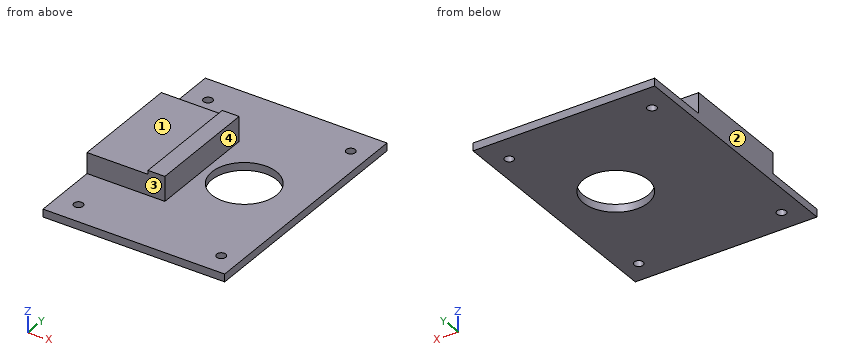
Autodesk Fusion 360 part; units mm, degrees
sketch "Sketch1" plane through (0, 0, 0) normal (0, 0, 1) x (1, 0, 0)
  line L0 (0, 0) -> (70, 0)
  line L1 (70, 0) -> (70, 54)
  line L2 (70, 54) -> (0, 54)
  line L3 (0, 54) -> (0, 0)
  line L4 (0, 0) -> (70, 0)
  line L5 (70, 0) -> (70, -20)
  line L6 (70, -20) -> (0, -20)
  line L7 (0, -20) -> (0, 0)
  line L8 (0, 54) -> (70, 54)
  line L9 (70, 54) -> (70, 74)
  line L10 (70, 74) -> (0, 74)
  line L11 (0, 74) -> (0, 54)
  dimension "d1" = 54
  dimension "d2" = 70
  dimension "d3" = 20
  dimension "d4" = 20
extrude "Extrude1" add sketch "Sketch1" along normal blind 3
hole "Hole1" at (45.2511, 28.5377, 3) direction (0, 0, -1) diameter 25 depth 5 tip angle 180
sketch "Sketch3" plane through (0, 0, 3) normal (0, 0, 1) x (-1, 0, 0)
  circle A0 centre (-45.2511, -28.5377) radius 12.5
  line L0 (0, -48.5) -> (-30.0019, -48.5)
  line L1 (-30.0019, -48.5) -> (-30.0019, -5.5)
  line L2 (-30.0019, -5.5) -> (0, -5.5)
  line L3 (0, -5.5) -> (0, -48.5)
  line L4 (-70, 20) -> (-70, -74)
  line L5 (-70, -74) -> (0, -74)
  line L6 (0, -74) -> (0, 20)
  line L7 (0, 20) -> (-70, 20)
  dimension "d20" = 25.5
  dimension "d21" = 25.5
extrude "Extrude3" add sketch "Sketch3" along normal blind 8 contours L0 L1 L2 L3 L6
sketch "Sketch4" plane through (0, 0, 3) normal (0, 0, 1) x (-1, 0, 0)
  line L0 (0, -48.5) -> (-30.0019, -48.5)
  line L1 (-30.0019, -48.5) -> (-30.0019, -5.5)
  line L2 (-30.0019, -5.5) -> (0, -5.5)
  line L3 (0, -5.5) -> (0, 20)
  line L4 (0, 20) -> (-70, 20)
  line L5 (-70, 20) -> (-70, -74)
  line L6 (-70, -74) -> (0, -74)
  line L7 (0, -74) -> (0, -48.5)
  circle A0 centre (-45.2511, -28.5377) radius 12.5
  circle A1 centre (-8, -63.531) radius 1.75
  circle A2 centre (-63, -63.531) radius 1.75
  circle A3 centre (-8, 11.469) radius 1.75
  circle A4 centre (-63, 11.469) radius 1.75
  dimension "d22" = 3.5
  dimension "d25" = -55
  dimension "d26" = 75
  dimension "d27" = 10.469
  dimension "d30" = 8
extrude "Extrude4" cut sketch "Sketch4" against normal blind 3 contours A1 | A2 | A3 | A4
sketch "Sketch5" plane through (0, 0, 11) normal (0, 0, 1) x (-1, 0, 0)
  line L0 (0, -5.5) -> (-30.0019, -5.5)
  line L1 (-30.0019, -5.5) -> (-30.0019, -48.5)
  line L2 (-30.0019, -48.5) -> (0, -48.5)
  line L3 (0, -48.5) -> (0, -5.5)
  line L4 (-30.0019, -5.5) -> (-23.4899, -5.5)
  line L5 (-23.4899, -5.5) -> (-23.4899, -48.5)
  line L6 (-23.4899, -48.5) -> (-30.0019, -48.5)
  line L7 (-30.0019, -48.5) -> (-30.0019, -5.5)
extrude "Extrude5" add sketch "Sketch5" along normal blind 1.5 contours L0 L1 L2 L4 L5 L6 L7
Geometry check sheet. Reference: the model listing, model coordinates, mm. Face numbers are marked on the shaded views. A direction names the side the tool comes from. Round coordinates to 2 decimals unless told otherwise and drop trailing zeros. Write each loop counter-clockwise with the first axis right and the second up, starting at its lowest first coordinate (ties: lowest second). Pieces come first, ordered by that corner, then holes. Notation, with made-up numbers: (4.5, 59) - (41.5, 59) arc R27 ccw to (41.5, 97) - close; hole circle Ø2 at (34.25, 78). An arc over 180 degrees is marked (long way). Write each question's results on one line, items separated by ' | '.
(1) Sectioned sample at A-A, the plane x = 63. Enter the section's corners in (y, z).
Computed:
outline: (-20, 0) - (-13.22, 0) - (-13.22, 3) - (-20, 3) - close; (-9.72, 0) - (61.78, 0) - (61.78, 3) - (-9.72, 3) - close; (65.28, 0) - (74, 0) - (74, 3) - (65.28, 3) - close
(2) Sectioned sample at B-B, the plane y = 40. Enter the section's corners in (x, z).
Computed:
outline: (0, 0) - (40.26, 0) - (40.26, 3) - (30, 3) - (30, 12.5) - (23.49, 12.5) - (23.49, 11) - (0, 11) - close; (50.24, 0) - (70, 0) - (70, 3) - (50.24, 3) - close
(3) Thickness scan on probe 1 along Y at (x, z) = (8, 2.4); probe 2 along Z at (x, y) = (59.5, -6); probe 3 along Z at (x, y) = (10, 48). Record the ranges inside material, lowest first. Write a range as from..to.
Computed:
probe 1: y = -20..-13.22, -9.72..61.78, 65.28..74 | probe 2: z = 0..3 | probe 3: z = 0..11
(4) Sectioned sample at D-D, the plane x = 36.5. Enter the section's corners in (y, z).
Computed:
outline: (-20, 0) - (19.61, 0) - (19.61, 3) - (-20, 3) - close; (37.46, 0) - (74, 0) - (74, 3) - (37.46, 3) - close
(5) Sectioned sample at C-C, the plane y = 8. Enter the section's corners in (x, z), plus the area to 3 significant figures.
Computed:
outline: (0, 0) - (70, 0) - (70, 3) - (30, 3) - (30, 12.5) - (23.49, 12.5) - (23.49, 11) - (0, 11) - close | area: 460 mm^2
(6) Depth check by flat-ended pin: pin 1 Ø1.2 at (y, z) = (18.5, 12) entering from -X; pin 2 Ø3 at (x, y) = (63, 63.531) entering from +Z; pin 3 Ø3 at (y, z) = (37, 6.5) entering from +X; pin 4 Ø7 at (x, y) = (15.5, 18.5) entering from +Z. Enter the tip coordinate at first touch or a pass-through.
Computed:
pin 1: stops at x = 23.49 | pin 2: passes through | pin 3: stops at x = 30 | pin 4: stops at z = 11
(7) Set-up check for the marked faces 1, 2, 3 and 4: record each of +Z, -Z, +X, -X, +Y, -Y from which the full face is reachable in a straight line by a thin tool's end or side.
Computed:
face 1: +Z, -X, +Y, -Y | face 2: +Z, -Z, -X, +Y, -Y | face 3: +Z, +X, -X, -Y | face 4: +Z, +X, +Y, -Y
